Autodesk Inventor part; units mm, degrees
ref_plane "YZ Plane" through (0, 0, 0) normal (1, 0, 0) x (0, 1, 0)
ref_plane "XZ Plane" through (0, 0, 0) normal (0, 1, 0) x (-1, 0, 0)
ref_plane "XY Plane" through (0, 0, 0) normal (0, 0, 1) x (1, 0, 0)
sketch "Sketch1" plane through (0, 0, 0) normal (0, 1, 0) x (-1, 0, 0)
  line L0 (0, 0) -> (10, 0)
  line L1 (10, 0) -> (10, -32)
  line L2 (10, -32) -> (0, -32)
  line L3 (0, -32) -> (0, 0)
  circle A0 centre (5, -6) radius 3.25
  circle A1 centre (5, -26) radius 3.25
  dimension "t" = 10
  dimension "d2" = 6.5
  dimension "d3" = 6.5
  dimension "d4" = 6
  dimension "d5" = 6
  dimension "d6" = 5
  dimension "d7" = 5
  dimension "height" = 32
extrude "Extrusion1" add sketch "Sketch1" along normal blind 14
sketch "Sketch2" plane through (0, 0, 0) normal (1, 0, 0) x (0, 0, -1)
  circle A0 centre (16, 7) radius 3.1
  line L0 (0, 0) -> (0, 14)
  line L1 (32, 0) -> (0, 0)
  dimension "d10" = 6.2
  dimension "d12" = 16
  dimension "d13" = 7
extrude "Extrusion2" cut sketch "Sketch2" against normal up to next
sketch "Sketch3" plane through (0, 0, 0) normal (1, 0, 0) x (0, 0, -1)
  circle A0 centre (16, 7) radius 3.1
  line L0 (22.0044, 7) -> (19.0022, 1.8)
  line L1 (19.0022, 1.8) -> (12.9978, 1.8)
  line L2 (12.9978, 1.8) -> (9.9956, 7)
  line L3 (9.9956, 7) -> (12.9978, 12.2)
  line L4 (12.9978, 12.2) -> (19.0022, 12.2)
  line L5 (19.0022, 12.2) -> (22.0044, 7)
  line L6 (0, 14) -> (32, 14)
  point P0 (0, 0)
  point P1 (16, 12.2)
  dimension "d16" = 10.4
extrude "Extrusion3" cut sketch "Sketch3" against normal blind 5
equation "\"d6\" = 0.5 * t"
equation "\"d7\" = 0.5 * t"
equation "\"d12\" = 0.5 * height"
properties part number "smallSprocketFixture" material "ABS Plastic"
CAD build for the part. Positions are in the model's coordinates, mm. A direction names the side the tool comes from. Round coordinates to 2 decimals unless told otherwise and drop trailing zeros. Loops run counter-clockwise (first coordinate to the right, second up) from the corner with the lowest first, then second, coordinate; pieces in that order, holes last. Notation, with made-up numbers: (5.25, -3) - (48.25, -3) arc R25 cw to (48.25, 13) - close; hole circle Ø10 at (-32.5, -21.5). An arc over 180 degrees is marked (long way). Return JSON: item names as keys, results as strings. Group by question number.
Q1. Two-plate mould, pull along Y, no slides. Class faces 3 (the face through (-5, 14, -16)), 4 (the face through (-2, 12.2, -16)), 5 (the face through (-8.1, 6.9, -6.98)): +Y half, -Y half, draft (parallel to the pull), parting line (faces both ways), or undercut.
Q2. Band-saw the part on C-C on x = -5.5. Give the cut face in (y, z), plus the area to 3 significant figures.
Q3. Band-saw the part on A-A on z = -6. Give the cut face in (x, y).
Q4. Tool access for faces 1 (the face through (-5, 7, 0)), 2 (the face through (-2.46, 4.36, -11.52)): list every direction of +Z, -Z, +X, -X, +Y, -Y with a clear straight run to the whole face (end or side of a thin tool).
Q5. Band-saw the part on D-D on y = 2.5. Give the cut face in (x, z).
Q6. Drill centre lines: line 1 along Y through (x, z) = (-1.25, -17.5); line 2 along Z through (x, y) = (-2.75, 10.5); line 3 along Z through (x, y) = (-5.75, 3). Where is each one in solid material? Low to high. Write a range as [from, to].
Q7. Band-saw the part on B-B on y = 8.25. Give the cut face in (x, z), plus the area to 3 significant figures.
Solutions:
{
 "1": {"face 3": "+Y half", "face 4": "undercut", "face 5": "draft"},
 "2": {"outline": "(0, -32) - (14, -32) - (14, -29.21) - (0, -29.21) - close; (0, -22.79) - (14, -22.79) - (14, -9.21) - (0, -9.21) - close; (0, -2.79) - (14, -2.79) - (14, 0) - (0, 0) - close; hole circle Ø6.2 at (7, -16)", "area": "238 mm^2"},
 "3": {"outline": "(-10, 0) - (-8.25, 0) - (-8.25, 14) - (-10, 14) - close; (-1.75, 0) - (0, 0) - (0, 14) - (-1.75, 14) - close"},
 "4": {"face 1": "+Z, +X, -X, +Y, -Y", "face 2": "+X"},
 "5": {"outline": "(-10, -32) - (0, -32) - (0, -19.41) - (-5, -19.41) - (-5, -12.59) - (0, -12.59) - (0, 0) - (-10, 0) - close; hole circle Ø6.5 at (-5, -26); hole circle Ø6.5 at (-5, -6)"},
 "6": {"line 1": "y = [0, 1.8], [12.2, 14]", "line 2": "z = [-32, -28.35], [-23.65, -19.98], [-12.02, -8.35], [-3.65, 0]", "line 3": "z = [-32, -29.16], [-22.84, -9.16], [-2.84, 0]"},
 "7": {"outline": "(-10, -32) - (0, -32) - (0, -21.28) - (-5, -21.28) - (-5, -18.84) - (-10, -18.84) - close; (-10, -13.16) - (-5, -13.16) - (-5, -10.72) - (0, -10.72) - (0, 0) - (-10, 0) - close; hole circle Ø6.5 at (-5, -26); hole circle Ø6.5 at (-5, -6)", "area": "172 mm^2"}
}
